Source: three-view drawing plus pictorial views. Frame: mm from the lowest corner of the part. A direction names the side the tool comes from. Give positions to 0.01 mm unless a question says otherwise; leave off trailing zeros. Write each loop counter-clockwise with the first axis right and the second up, starting at its lowest first coordinate (ties: lowest second). Pieces come first, ordered by that corner, then holes. Notation, with made-up numbers: (-16, 83) -> (35, 83) arc R23 cw to (35, 106) -> close; hole circle Ø2 at (51.5, -37). An arc over 180 degrees is marked (long way). Answer in a Markdown table with one row per item. Add a question column.
Item 1: Section query B-B on y = 16. Output: boundary loops of the cut face in (x, z).
Item 2: Section query D-D on x = 7.5. Output: boundary loops of the cut face in (y, z).
Item 3: First-contact query: P1, Ø3, axis at y = 4, z = 4, coming from the +X side; P2, Ø3.5, axis at y = 16, z = 4, coming from the +X side. Flat tips, straight axial feed; report the tip coordinate or a pass-through.
Item 4: Material intervals for probe 1 along Y at (x, z) = (7.3, 4); probe 2 along Y at (x, z) = (6.1, 4) (1 decimal); probe 3 along Y at (x, z) = (5.7, 4) (1 decimal), sorted ascending. Write a range as from..to.
Item 5: Access query for the marked faces 1, 2 and 3. Directions: +Z, -Z, +X, -X, +Y, -Y. A direction counts if a zero-diameter tool reaches every point of the face in a straight line with its end or side. Return the directions, or none.
Item 6: Draft query along Z for the marked faces 4, 5, 6 and 7. Return one class per face: +Z half, -Z half, draft (parallel to the pull), parting line (faces both ways), or undercut.
Item 7: Section query C-C on z = 4.5. State how many separate pieces and enclosed holes the cut face has.
Item 8: Section query A-A on x = 4. Output: boundary loops of the cut face in (y, z).
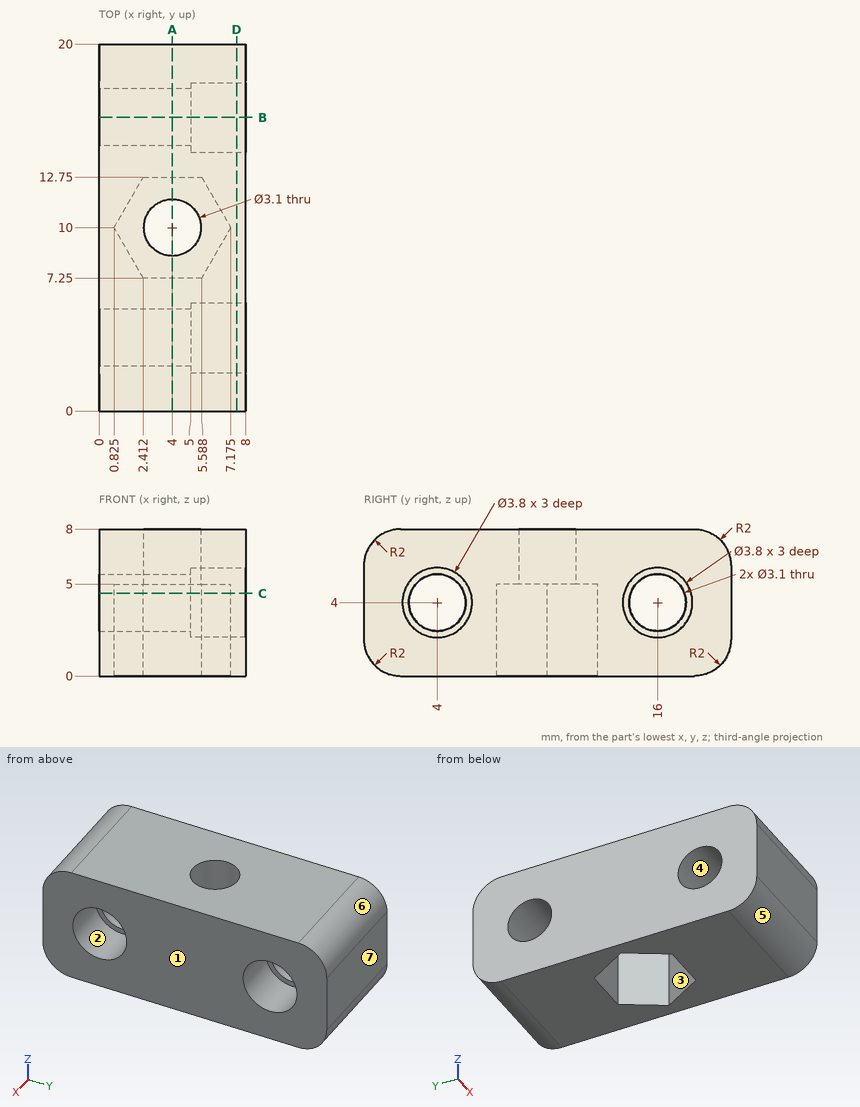
Findings below:
| question | item | result |
|---|---|---|
| 1 | outline | (0, 0) -> (8, 0) -> (8, 2.1) -> (5, 2.1) -> (5, 2.45) -> (0, 2.45) -> close; (0, 5.55) -> (5, 5.55) -> (5, 5.9) -> (8, 5.9) -> (8, 8) -> (0, 8) -> close |
| 2 | outline | (0, 2) arc R2 ccw to (2, 0) -> (18, 0) arc R2 ccw to (20, 2) -> (20, 6) arc R2 ccw to (18, 8) -> (2, 8) arc R2 ccw to (0, 6) -> close; hole circle Ø3.8 at (4, 4); hole circle Ø3.8 at (16, 4) |
| 3 | P1 | passes through |
| 3 | P2 | stops at x = 5 |
| 4 | probe 1 | y = 0..2.1, 5.9..14.1, 17.9..20 |
| 4 | probe 2 | y = 0..2.1, 5.9..8.1, 11.9..14.1, 17.9..20 |
| 4 | probe 3 | y = 0..2.1, 5.9..7.4, 12.6..14.1, 17.9..20 |
| 5 | face 1 | +Z, -Z, +X, +Y, -Y |
| 5 | face 2 | +X |
| 5 | face 3 | -Z |
| 6 | face 4 | undercut |
| 6 | face 5 | -Z half |
| 6 | face 6 | +Z half |
| 6 | face 7 | draft |
| 7 | separate pieces | 3 |
| 7 | enclosed holes | 1 |
| 8 | outline | (0, 2) arc R2 ccw to (2, 0) -> (7.25, 0) -> (7.25, 5) -> (8.45, 5) -> (8.45, 8) -> (2, 8) arc R2 ccw to (0, 6) -> close; (11.55, 5) -> (12.75, 5) -> (12.75, 0) -> (18, 0) arc R2 ccw to (20, 2) -> (20, 6) arc R2 ccw to (18, 8) -> (11.55, 8) -> close; hole circle Ø3.1 at (4, 4); hole circle Ø3.1 at (16, 4) |
